Verification items for the finished model (mm, model axes). Face numbers are marked on the shaded views. A direction names the side the tool comes from. Give positions to 0.01 mm unless a question says otherwise; leave off trailing zeros. Loops run counter-clockwise (first coordinate to the right, second up) from the corner with the lowest first, then second, coordinate; pieces in that order, holes last. Notation, with made-up numbers: M 65.5,-29.5 L 120.5,-29.5 A18 ccw 120.5,1.5 Z; hole C 65,26 d10. An arc over 180 degrees is marked long. Use CSV: the item, a comma, the result in double quotes.
from build123d import *

# Parameters (mm, degrees)
BOSS_EXTRU_1_DEPTH           = 20
CONG_1_R                     = 10
CONG_2_R                     = 10
ESQUISSE3_R                  = 2.5
ENL_V_MAT_EXTRU_1_DEPTH      = 20
ESQUISSE4_R                  = 2.5
ENL_V_MAT_EXTRU_2_DEPTH      = 106
ESQUISSE5_R                  = 4.2
ENL_V_MAT_EXTRU_3_DEPTH      = 3
ENL_V_MAT_EXTRU_3_DEPTH_BACK = 13


with BuildPart() as part:
    # Esquisse2 → Boss.-Extru.1 (new body)
    with BuildSketch(Plane.XY):
        with BuildLine():
            Line((0, 0), (45, 0))
            Line((45, 0), (45, -100))
            Line((45, -100), (65, -100))
            ThreePointArc((65, -100), (83.49592747, -46.791003359), (130, -15))
            Line((130, -15), (130, 5))
            Line((130, 5), (0, 5))
            Line((0, 5), (0, 0))
        make_face()
        with BuildLine():
            Line((115, -5), (55, -5))
            Line((55, -5), (55, -71.357566363))
            ThreePointArc((55, -71.357566363), (77.53382116, -31.427921826), (115, -5))
        make_face(mode=Mode.SUBTRACT)
    extrude(amount=BOSS_EXTRU_1_DEPTH)

    # Congé1
    cong_1_edges = [part.edges().sort_by_distance(p)[0] for p in [
        (130, -15, 10),
    ]]
    fillet(cong_1_edges, radius=CONG_1_R)

    # Congé2
    cong_2_edges = [part.edges().sort_by_distance(p)[0] for p in [
        (65, -100, 10),
    ]]
    fillet(cong_2_edges, radius=CONG_2_R)

    # Esquisse3 → Enlèv. mat.-Extru.1 (cut)
    with BuildSketch(Plane.XZ):
        with Locations((33.75, 10)):
            Circle(ESQUISSE3_R)
        with Locations((11.25, 10)):
            Circle(ESQUISSE3_R)
    extrude(amount=-ENL_V_MAT_EXTRU_1_DEPTH, mode=Mode.SUBTRACT)

    # Esquisse4 → Enlèv. mat.-Extru.2 (cut, through all)
    with BuildSketch(Plane(origin=(0, 5, 0), x_dir=(1, 0, 0), z_dir=(0, 1, 0))):
        with Locations((120, -10)):
            Circle(ESQUISSE4_R)
    extrude(amount=-ENL_V_MAT_EXTRU_2_DEPTH, mode=Mode.SUBTRACT)

    # Esquisse5 → Enlèv. mat.-Extru.3 (cut, two sides)
    with BuildSketch(Plane(origin=(0, -17.190046968, 0), x_dir=(1, 0, 0), z_dir=(0, 1, 0))) as enl_v_mat_extru_3_sk:
        with Locations((120, -10)):
            Circle(ESQUISSE5_R)
    extrude(amount=ENL_V_MAT_EXTRU_3_DEPTH, mode=Mode.SUBTRACT)
    extrude(enl_v_mat_extru_3_sk.sketch, amount=-ENL_V_MAT_EXTRU_3_DEPTH_BACK, mode=Mode.SUBTRACT)


solid = part.part
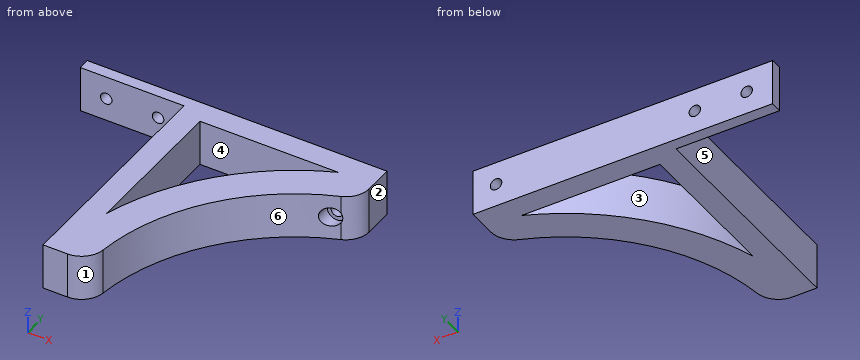
(1) Section check C-C on z = 4. Record the cut outline in (x, y).
Calculated:
outline,"M 0,0 L 45,0 L 45,-100 L 55.65,-100 A10 ccw 65.58,-91.15 A90 cw 123.5,-17.15 A10 ccw 130,-7.78 L 130,5 L 0,5 Z; hole M 55,-71.36 A104.42 cw 115,-5 L 55,-5 Z"
(2) Depth check by flat-ended pin: pin 1 Ø6 at (x, z) = (31.5, 11) entering from -Y; pin 2 Ø5 at (y, z) = (-40, 13.5) entering from +X; pin 3 Ø4 at (x, z) = (92, 17.5) entering from -Y; pin 4 Ø1.5 at (x, y) = (51, -79) entering from -Z. Enter the tip coordinate at first touch or a pass-through.
Calculated:
pin 1,"stops at y = 0"
pin 2,"stops at x = 91.67"
pin 3,"stops at y = -39.2"
pin 4,"stops at z = 0"
(3) Scan lines: L1, parallel to Z at x = 120, y = -16; L2, parallel to Z at x = 120, y = 0; L3, parallel to X at y = -4, z = 10. Record each from-to range of solid material in increasing order. Write a range as from..to.
Calculated:
L1,"z = 0..5.8, 14.2..20"
L2,"z = 0..7.5, 12.5..20"
L3,"x = 45..117.5, 122.5..130"
(4) Section check D-D on y = -58.5. Record the cut outline in (x, z), plus the area to 3 significant figures.
Calculated:
outline,"M 45,0 L 55,0 L 55,20 L 45,20 Z; M 59.81,0 L 75.9,0 L 75.9,20 L 59.81,20 Z"
area,"522 mm²"
(5) Section check B-B on z = 10. Record the cut outline in (x, y), plus the area to 3 significant figures.
Calculated:
outline,"M 0,0 L 8.75,0 L 8.75,5 L 0,5 Z; M 13.75,0 L 31.25,0 L 31.25,5 L 13.75,5 Z; M 36.25,0 L 45,0 L 45,-100 L 55.65,-100 A10 ccw 65.58,-91.15 A90 cw 115.8,-20.44 L 115.8,-14.19 L 117.5,-14.19 L 117.5,5 L 36.25,5 Z; M 122.5,-14.19 L 124.2,-14.19 L 124.2,-16.86 A10 ccw 130,-7.78 L 130,5 L 122.5,5 Z; hole M 55,-71.36 A104.42 cw 115,-5 L 55,-5 Z"
area,"3,510 mm²"
(6) Section check A-A on x = 33.75. Record the cut outline in (y, z).
Calculated:
outline,"M 0,0 L 5,0 L 5,7.5 L 0,7.5 Z; M 0,12.5 L 5,12.5 L 5,20 L 0,20 Z"
(7) Tool access check on the marked faces 4, 5 and 6. Record the directions out of +Z, -Z, +X, -X, +Y, -Y that give a thin tool (end or side, any length) a straight path to the whole face; none if there is none.
Calculated:
face 4,"+Z, -Z"
face 5,"+Z, -Z, -X, -Y"
face 6,"+Z, -Z, +X, -Y"
(8) Mould release check, pull along Y, two halves, no side actions. Record for the marked faces 1, 2 and 3: released by +Y, released by -Y, zero draft, split by the parting line, or undercut.
Calculated:
face 1,"released by -Y"
face 2,"zero draft"
face 3,"undercut"
